Geometry: final body of the model. Coordinates: model frame, mm. A direction names the side the tool comes from. Give positions to 0.01 mm unless a question says otherwise; leave off trailing zeros. Loops run counter-clockwise (first coordinate to the right, second up) from the corner with the lowest first, then second, coordinate; pieces in that order, holes last. Notation, with made-up numbers: (77, 79) -> (122, 79) arc R26 cw to (122, 103) -> close; hole circle Ø7 at (2.25, 39). An arc over 180 degrees is marked (long way). Answer in a Markdown table with one row per item. Add a question column.
1) Line query: line 1 (X direction, y = 3.6, z = -67); line 2 (Z direction, x = -3, y = 1.8); line 3 (X direction, y = 0.6, z = -67.5). Output: solid intervals per line, ascending. Write a range as from..to.
2) Section query B-B (z = 57). Return the cut outline in (x, y).
3) First-contact query: P1, Ø3.5, axis at x = 45.25, z = 45.25, coming from the -Y side; P2, Ø2, axis at x = 0.5, y = 1, coming from the -Z side; P3, Ø1.2, axis at x = -81, y = 2.5, coming from the -Z side. Flat tips, straight axial feed; report the tip coordinate or a pass-through.
4) Section query A-A (y = 1.8). Return the cut outline in (x, z), plus the area to 3 significant figures.
5) Access query for faces 5 (the flat face through (-78, 2, -22.5)), 6 (the flat face through (78, 2, -22.5)), 7 (the flat face through (-78, 2, 22.5)), 8 (the flat face through (12.5, 2, -64)). Directions: +Z, -Z, +X, -X, +Y, -Y. A direction counts if a zero-diameter tool reaches every point of the face in a straight line with its end or side. Return the directions, or none.
6) Section query C-C (x = 75). Return the cut outline in (y, z), plus the area to 3 significant figures.
7) Draft query along X for faces 1 (the cylindrical face through (-48.84, 1.97, 56.92)), 2 (the cylindrical face through (44.994, 2.028, 43.272)), 3 (the flat face through (85, 2, 0)), 4 (the flat face through (1, 0, 1)). Return one class per face: +X half, -X half, draft (parallel to the pull), parting line (faces both ways), or undercut.
8) Section query D-D (z = -63). Return the cut outline in (x, y).
Autodesk Inventor part; units mm, degrees
ref_plane "YZ Plane" through (0, 0, 0) normal (1, 0, 0) x (0, 1, 0)
ref_plane "XZ Plane" through (0, 0, 0) normal (0, 1, 0) x (-1, 0, 0)
ref_plane "XY Plane" through (0, 0, 0) normal (0, 0, 1) x (1, 0, 0)
sketch "Boceto1" plane through (0, 0, 0) normal (0, 1, 0) x (-1, 0, 0)
  line L0 (0, -55) -> (12.5, -55)
  line L1 (12.5, -55) -> (12.5, -73.951)
  line L2 (0, -55) -> (-12.5, -55)
  line L3 (-12.5, -55) -> (-12.5, -73.951)
  line L4 (0, 55) -> (12.5, 55)
  line L5 (12.5, 55) -> (12.5, 73.951)
  line L6 (0, 55) -> (-12.5, 55)
  line L7 (-12.5, 55) -> (-12.5, 73.951)
  line L8 (85, 0) -> (85, -22.5)
  line L9 (85, -22.5) -> (71.5454, -22.5)
  line L10 (85, 0) -> (85, 22.5)
  line L11 (85, 22.5) -> (71.5454, 22.5)
  line L12 (-85, 0) -> (-85, -22.5)
  line L13 (-85, -22.5) -> (-71.5454, -22.5)
  line L14 (-85, 0) -> (-85, 22.5)
  line L15 (-85, 22.5) -> (-71.5454, 22.5)
  arc A0 (12.5, -73.951) -> (71.5454, -22.5) centre (0, 0) ccw
  arc A1 (71.5454, 22.5) -> (12.5, 73.951) centre (0, 0) ccw
  arc A2 (-12.5, 73.951) -> (-71.5454, 22.5) centre (0, 0) ccw
  arc A3 (-71.5454, -22.5) -> (-12.5, -73.951) centre (0, 0) ccw
  dimension "d2" = 12.5
  dimension "d4" = 22.5
extrude "Extrusión1" add sketch "Boceto1" along normal blind 4
sketch "Boceto2" plane through (0, 4, 0) normal (0, 1, 0) x (1, 0, 0)
  circle A0 centre (0, 0) radius 64
  line L0 (0, 0) -> (64, 0) construction
  circle A1 centre (45.2548, 45.2548) radius 2
  circle A2 centre (-45.2548, 45.2548) radius 2
  circle A3 centre (-45.2548, -45.2548) radius 2
  circle A4 centre (45.2548, -45.2548) radius 2
  dimension "d9" = 4
  dimension "d12" = 360
extrude "Extrusión2" cut sketch "Boceto2" against normal blind 4 contours A1 A0 | A0 A1 | A4 A0 | A0 A4 | A2 A0 | A0 A2 | A3 A0 | A0 A3
properties part number "Base_inferior"
Evaluation:
| question | item | result |
|---|---|---|
| 1 | line 1 | -33.7..-12.5, 12.5..33.7 |
| 1 | line 2 | -55..55 |
| 1 | line 3 | -32.69..-12.5, 12.5..32.69 |
| 2 | outline | (-48.74, 0) -> (-12.5, 0) -> (-12.5, 4) -> (-48.74, 4) -> close; (12.5, 0) -> (48.74, 0) -> (48.74, 4) -> (12.5, 4) -> close |
| 3 | P1 | through |
| 3 | P2 | z = -55 |
| 3 | P3 | z = -22.5 |
| 4 | outline | (-85, -22.5) -> (-71.55, -22.5) arc R75 ccw to (-12.5, -73.95) -> (-12.5, -55) -> (12.5, -55) -> (12.5, -73.95) arc R75 ccw to (71.55, -22.5) -> (85, -22.5) -> (85, 22.5) -> (71.55, 22.5) arc R75 ccw to (12.5, 73.95) -> (12.5, 55) -> (-12.5, 55) -> (-12.5, 73.95) arc R75 ccw to (-71.55, 22.5) -> (-85, 22.5) -> close; hole circle Ø4 at (-45.25, -45.25); hole circle Ø4 at (-45.25, 45.25); hole circle Ø4 at (45.25, -45.25); hole circle Ø4 at (45.25, 45.25) |
| 4 | area | 17,600 mm² |
| 5 | face 5 | -Z, -X, +Y, -Y |
| 5 | face 6 | -Z, +X, +Y, -Y |
| 5 | face 7 | +Z, -X, +Y, -Y |
| 5 | face 8 | -Z, +Y, -Y |
| 6 | outline | (0, -22.5) -> (4, -22.5) -> (4, 22.5) -> (0, 22.5) -> close |
| 6 | area | 180 mm² |
| 7 | face 1 | -X half |
| 7 | face 2 | undercut |
| 7 | face 3 | +X half |
| 7 | face 4 | draft |
| 8 | outline | (-40.69, 0) -> (-12.5, 0) -> (-12.5, 4) -> (-40.69, 4) -> close; (12.5, 0) -> (40.69, 0) -> (40.69, 4) -> (12.5, 4) -> close |
